Design review of the part built by this model. Coordinates are the model's own, in mm. Give positions to 0.01 mm unless a question says otherwise; leave off trailing zeros. Loops run counter-clockwise (first coordinate to the right, second up) from the corner with the lowest first, then second, coordinate; pieces in that order, holes last. Notation, with made-up numbers: M -8,39.5 L 30,39.5 A7 cw 30,44.5 Z; hole C 25.25,-28.5 d1. An arc over 180 degrees is marked long. Use a Markdown table: item, result. Add a question column.
(1) Draft analysis for pull direction Y (two halves, no side actions). For faces 1 (the face through (2, -50, -1)), 2 (the face through (2, 50, 1)), 3 (the face through (2, 1, -51)), 4 (the face through (1, -2, 12)), state which applies: pulls with the +Y half, pulls with the -Y half, needs draft (parallel to the pull), parting line crosses it, or undercut.
(2) Insertion check: pin 1 Ø5 at (y, z) = (0, -12) entering from -X. The pin has a flat end and moves straight along its axis. Give the tip position at first contact, or say it passes through.
(3) Add section A-A, the plane y = 12. Give the boundary of the cut face in (x, z).
(4) For probe 1 along Z at (x, y) = (3.05, -12); probe 2 along Y at (x, z) = (3.6, 12); probe 3 along Z at (x, y) = (2.8, 38.1), list the stretches that pass through material, from the lowest coordinate up.
(5) Add section C-C, the plane y = 38.1. Give the boundary of the cut face in (x, z), then the cut area to 3 significant figures.
(6) Add section B-B, the plane z = -12. Give the boundary of the cut face in (x, y), then the cut area to 3 significant figures.
Autodesk Inventor part; units mm, degrees
ref_plane "YZ Plane" through (0, 0, 0) normal (1, 0, 0) x (0, 1, 0)
ref_plane "XZ Plane" through (0, 0, 0) normal (0, 1, 0) x (-1, 0, 0)
ref_plane "XY Plane" through (0, 0, 0) normal (0, 0, 1) x (1, 0, 0)
sketch "Sketch1" plane through (0, 0, 0) normal (1, 0, 0) x (0, 1, 0)
  point P0 (0, 0)
  point P1 (0, 12)
  dimension "d0" = 12
sketch "Sketch2" plane through (0, 0, 0) normal (1, 0, 0) x (0, 1, 0)
  line L0 (-50, 51) -> (50, 51)
  line L1 (50, 51) -> (50, -51)
  line L2 (50, -51) -> (-50, -51)
  line L3 (-50, -51) -> (-50, 51)
  line L4 (-50, 51) -> (50, -51) construction
  line L5 (50, 51) -> (-50, -51) construction
  point P0 (0, 0)
  dimension "d1" = 100
  dimension "d2" = 102
extrude "Extrusion1" add sketch "Sketch2" along normal blind 5
hole "Hole1" at (0, 0, 12) direction (1, 0, 0) diameter 3.2 end through all countersink diameter 6 countersink angle 90
pattern_circular "Circular Pattern1" count 4 over 360 about axis through (-10, 0, 0) along (1, 0, 0) of "Hole1"
sketch "Sketch3" plane through (0, 0, 0) normal (-1, 0, 0) x (0, 0, 1)
  point P0 (0, 0)
  point P1 (0, 38.1)
  point P2 (0, -38.1)
  dimension "d15" = 38.1
  dimension "d16" = 38.1
hole "Hole2" at (0, -38.1, 0) at (0, 38.1, 0) direction (1, 0, 0) diameter 6.647 end through all
chamfer "Chamfer1" distance 1 angle 45 12 edges at (0, 0, -51) (0, -50, 0) (0, 0, 51) (0, 50, 0) (2.5, 50, 51) (5, 0, 51) (2.5, -50, 51) (5, -50, 0) (2.5, -50, -51) (5, 0, -51) (2.5, 50, -51) (5, 50, 0)
sketch "Sketch4" plane through (0, 0, 0) normal (-1, 0, 0) x (0, 0, 1)
  point P0 (0, 0)
  point P1 (0, 0)
hole "Hole3" at (0, 0, 0) direction (1, 0, 0) diameter 12 depth 10 tip angle 118
chamfer "Chamfer3" distance 0.2 angle 45 4 edges at (0, -38.1, -3.3235) (0, 38.1, -3.3235) (5, -38.1, -3.3235) (5, 38.1, -3.3235)
chamfer "Chamfer4" distance 0.3 angle 45 2 edges at (0, 0, -6) (5, 0, -6)
properties part number "plytkaadaptacyjna" material "Stainless Steel"
Established:
| question | item | result |
|---|---|---|
| 1 | face 1 | pulls with the -Y half |
| 1 | face 2 | pulls with the +Y half |
| 1 | face 3 | needs draft |
| 1 | face 4 | undercut |
| 2 | pin 1 | x = 0.5 |
| 3 | outline | M 0,-50 L 1,-51 L 4,-51 L 5,-50 L 5,-1.6 L 1.4,-1.6 L 0,-3 Z; M 0,3 L 1.4,1.6 L 5,1.6 L 5,50 L 4,51 L 1,51 L 0,50 Z |
| 4 | probe 1 | -51 to -1.6, 1.6 to 51 |
| 4 | probe 2 | -50 to -1.6, 1.6 to 50 |
| 4 | probe 3 | -51 to -3.32, 3.32 to 51 |
| 5 | outline | M 0,-50 L 1,-51 L 4,-51 L 5,-50 L 5,-3.52 L 4.8,-3.32 L 0.2,-3.32 L 0,-3.52 Z; M 0,3.52 L 0.2,3.32 L 4.8,3.32 L 5,3.52 L 5,50 L 4,51 L 1,51 L 0,50 Z |
| 5 | area | 475 mm^2 |
| 6 | outline | M 0,-49 L 1,-50 L 4,-50 L 5,-49 L 5,-1.6 L 1.4,-1.6 L 0,-3 Z; M 0,3 L 1.4,1.6 L 5,1.6 L 5,49 L 4,50 L 1,50 L 0,49 Z |
| 6 | area | 480 mm^2 |
